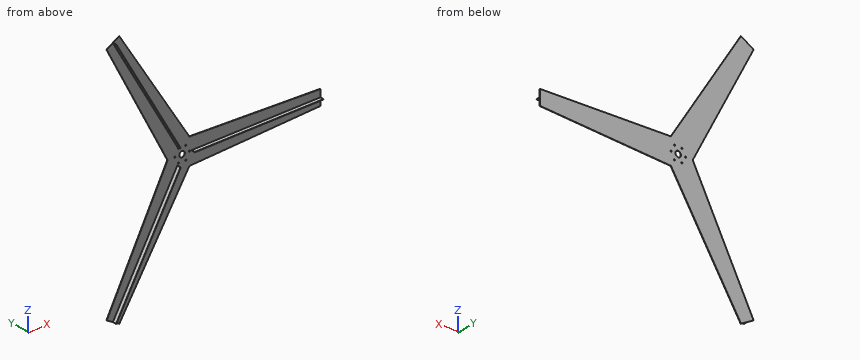
```python
from build123d import *

# Parameters (mm, degrees)
CROQUIS1_R              = 19.05
SALIENTE_EXTRUIR3_DEPTH = 2.5
CROQUIS2_W              = 885
CROQUIS2_H              = 2.5
SALIENTE_EXTRUIR4_DEPTH = 25.4
CROQUIS4_R              = 4
CORTAR_EXTRUIR1_DEPTH   = 2.54


with BuildPart() as part:
    # Croquis1 → Saliente-Extruir3 (new body)
    with BuildSketch(Plane(origin=(0, 0, 0), x_dir=(1, 0, 0), z_dir=(0, 1, 0))):
        Polygon((-431.698729811, -847.724133595), (-518.301270189, -797.724133595), (-100, 0), (-518.301270189, 797.724133595), (-431.698729811, 847.724133595), (50, 86.602540378), (950, 50), (950, -50), (50, -86.602540378), align=None)
        Circle(CROQUIS1_R, mode=Mode.SUBTRACT)
    extrude(amount=SALIENTE_EXTRUIR3_DEPTH)

    # Croquis2 → Saliente-Extruir4 (add)
    with BuildSketch(Plane.XZ):
        with Locations((507.5, 0)):
            Rectangle(CROQUIS2_W, CROQUIS2_H)
        Polygon((-473.917468245, -823.349133595), (-31.417468245, -56.916651246), (-33.582531755, -55.666651246), (-476.082531755, -822.099133595), align=None)
        Polygon((-476.082531755, 822.099133595), (-33.582531755, 55.666651246), (-31.417468245, 56.916651246), (-473.917468245, 823.349133595), align=None)
    extrude(amount=SALIENTE_EXTRUIR4_DEPTH)

    # Croquis4 → Cortar-Extruir1 (cut)
    with BuildSketch(Plane(origin=(0, 2.5, 0), x_dir=(1, 0, 0), z_dir=(0, 1, 0))):
        with Locations((25, -43.301270189)):
            Circle(CROQUIS4_R)
        with Locations((-25, -43.301270189)):
            Circle(CROQUIS4_R)
        with Locations((-50, 0)):
            Circle(CROQUIS4_R)
        with Locations((-25, 43.301270189)):
            Circle(CROQUIS4_R)
        with Locations((25, 43.301270189)):
            Circle(CROQUIS4_R)
        with Locations((50, 0)):
            Circle(CROQUIS4_R)
    extrude(amount=-CORTAR_EXTRUIR1_DEPTH, mode=Mode.SUBTRACT)


solid = part.part
```
Work out the finished part from the listing and answer in its coordinate system (mm). Give positions to 0.01 mm unless a question says otherwise; leave off trailing zeros. Write each loop counter-clockwise with the first axis right and the second up, starting at its lowest first coordinate (ties: lowest second). Pieces come first, ordered by that corner, then holes.
(1) Straight lines are drawn through the part: line 1 (X direction, y = 1.15, z = 0); line 2 (Z direction, x = -25, y = 0.6); line 3 (Y direction, x = -276.5, z = -541.5). For each, find the intervals that lie inside material, in ascending order.
Final values:
line 1: x = -100 to -54, -46 to -19.05, 19.05 to 46, 54 to 950
line 2: z = -205.11 to -47.3, -39.3 to 39.3, 47.3 to 205.11
line 3: y = 0 to 2.5
(2) The part is cut by section C-C on z = 668.5. Write down the section's boundary in (x, y), plus the area to 3 significant figures.
Final values:
outline: (-450.54, 0) - (-387.4, 0) - (-387.4, -25.4) - (-384.52, -25.4) - (-384.52, 0) - (-318.27, 0) - (-318.27, 2.5) - (-450.54, 2.5) - close
area: 404 mm2
(3) The part is cut by section B-B on x = 0. Write down the section's boundary in (y, z), plus the area to 3 significant figures.
Final values:
outline: (0, -165.61) - (2.5, -165.61) - (2.5, -19.05) - (0, -19.05) - close; (0, 19.05) - (2.5, 19.05) - (2.5, 165.61) - (0, 165.61) - close
area: 733 mm2
(4) Flat-ended cylindrical pins translate along their axes: pin 1 Ø1 at (y, z) = (-14.5, -310.5) entering from -X; pin 2 Ø10 at (y, z) = (-6.5, -61) entering from +X; pin 3 Ø7.5 at (x, y) = (516.5, -14.5) entering from -Z; pin 4 Ø13 at (x, z) = (25, -43.3) entering from +Y. Find the tip coordinate at first contact, or state that the pin passes through.
Final values:
pin 1: stops at x = -181
pin 2: stops at x = -31.42
pin 3: stops at z = -1.25
pin 4: stops at y = 2.5
(5) The part is cut by section A-A on y = -17. Write down the section's boundary in (x, z).
Final values:
outline: (-476.08, -822.1) - (-473.92, -823.35) - (-31.42, -56.92) - (-33.58, -55.67) - close; (-476.08, 822.1) - (-33.58, 55.67) - (-31.42, 56.92) - (-473.92, 823.35) - close; (65, -1.25) - (950, -1.25) - (950, 1.25) - (65, 1.25) - close
(6) The part is cut by section D-D on x = 841. Write down the section's boundary in (y, z), plus the area to 3 significant figures.
Final values:
outline: (-25.4, -1.25) - (0, -1.25) - (0, -54.43) - (2.5, -54.43) - (2.5, 54.43) - (0, 54.43) - (0, 1.25) - (-25.4, 1.25) - close
area: 336 mm2
